```python
from build123d import *

# Parameters (mm, degrees)
SKETCH1_R           = 2.5
BOSS_EXTRUDE1_DEPTH = 10
FILLET1_R           = 20
FILLET2_R           = 2.5


with BuildPart() as part:
    # Sketch1 → Boss-Extrude1 (new body)
    with BuildSketch(Plane(origin=(0, 0, 0), x_dir=(1, 0, 0), z_dir=(0, 1, 0))):
        with BuildLine():
            Line((0, 0), (-300, 0))
            Line((-300, 0), (-300, 125))
            Line((-300, 125), (-287.5, 155))
            Line((-287.5, 155), (-275, 125))
            Line((-275, 125), (-275, 97))
            Line((-275, 97), (-287.66515139, 62))
            ThreePointArc((-287.66515139, 62), (-280.543096437, 48.210936871), (-268.5, 58))
            Line((-268.5, 58), (-268.5, 83))
            ThreePointArc((-268.5, 83), (-262.136038969, 80.363961031), (-259.5, 74))
            Line((-259.5, 74), (-259.5, 25))
            Line((-259.5, 25), (-248.5, 25))
            Line((-248.5, 25), (-248.5, 86.008335649))
            ThreePointArc((-248.5, 86.008335649), (-262.197622342, 96.159801673), (-257.553360344, 112.564311745))
            Line((-257.553360344, 112.564311745), (-242.5, 125))
            Line((-242.5, 125), (-230, 155))
            Line((-230, 155), (-217.5, 125))
            Line((-217.5, 125), (-217.5, 97))
            Line((-217.5, 97), (-230.16515139, 62))
            ThreePointArc((-230.16515139, 62), (-223.043096437, 48.210936871), (-211, 58))
            Line((-211, 58), (-211, 83))
            ThreePointArc((-211, 83), (-204.636038969, 80.363961031), (-202, 74))
            Line((-202, 74), (-202, 25))
            Line((-202, 25), (-191, 25))
            Line((-191, 25), (-191, 86.008335649))
            ThreePointArc((-191, 86.008335649), (-204.697622342, 96.159801673), (-200.053360344, 112.564311745))
            Line((-200.053360344, 112.564311745), (-185, 125))
            Line((-185, 125), (-172.5, 155))
            Line((-172.5, 155), (-160, 125))
            Line((-160, 125), (-160, 97))
            Line((-160, 97), (-172.66515139, 62))
            ThreePointArc((-172.66515139, 62), (-165.543096437, 48.210936871), (-153.5, 58))
            Line((-153.5, 58), (-153.5, 83))
            ThreePointArc((-153.5, 83), (-147.136038969, 80.363961031), (-144.5, 74))
            Line((-144.5, 74), (-144.5, 25))
            Line((-144.5, 25), (-133.5, 25))
            Line((-133.5, 25), (-133.5, 86.008335649))
            ThreePointArc((-133.5, 86.008335649), (-147.197622342, 96.159801673), (-142.553360344, 112.564311745))
            Line((-142.553360344, 112.564311745), (-127.5, 125))
            Line((-127.5, 125), (-115, 155))
            Line((-115, 155), (-102.5, 125))
            Line((-102.5, 125), (-102.5, 97))
            Line((-102.5, 97), (-115.16515139, 62))
            ThreePointArc((-115.16515139, 62), (-108.043096437, 48.210936871), (-96, 58))
            Line((-96, 58), (-96, 83))
            ThreePointArc((-96, 83), (-89.636038969, 80.363961031), (-87, 74))
            Line((-87, 74), (-87, 25))
            Line((-87, 25), (-76, 25))
            Line((-76, 25), (-76, 86.008335649))
            ThreePointArc((-76, 86.008335649), (-89.697622342, 96.159801673), (-85.053360344, 112.564311745))
            Line((-85.053360344, 112.564311745), (-70, 125))
            Line((-70, 125), (-57.5, 155))
            Line((-57.5, 155), (-45, 125))
            Line((-45, 125), (-45, 97))
            Line((-45, 97), (-57.66515139, 62))
            ThreePointArc((-57.66515139, 62), (-50.543096437, 48.210936871), (-38.5, 58))
            Line((-38.5, 58), (-38.5, 83))
            ThreePointArc((-38.5, 83), (-32.136038969, 80.363961031), (-29.5, 74))
            Line((-29.5, 74), (-29.5, 25))
            Line((-29.5, 25), (-18.5, 25))
            Line((-18.5, 25), (-18.5, 86.008335649))
            ThreePointArc((-18.5, 86.008335649), (-32.197622342, 96.159801673), (-27.553360344, 112.564311745))
            Line((-27.553360344, 112.564311745), (-12.5, 125))
            Line((-12.5, 125), (0, 155))
            Line((0, 155), (0, 0))
        make_face()
        with Locations(Location((-5, 125, 0), (0, 0, 270))):
            Circle(SKETCH1_R, mode=Mode.SUBTRACT)
        with Locations(Location((-58.5, 87, 0), (0, 0, 270))):
            Circle(SKETCH1_R, mode=Mode.SUBTRACT)
        with Locations(Location((-62.5, 125, 0), (0, 0, 270))):
            Circle(SKETCH1_R, mode=Mode.SUBTRACT)
        with Locations(Location((-116, 87, 0), (0, 0, 270))):
            Circle(SKETCH1_R, mode=Mode.SUBTRACT)
        with Locations(Location((-120, 125, 0), (0, 0, 270))):
            Circle(SKETCH1_R, mode=Mode.SUBTRACT)
        with Locations(Location((-173.5, 87, 0), (0, 0, 270))):
            Circle(SKETCH1_R, mode=Mode.SUBTRACT)
        with Locations(Location((-177.5, 125, 0), (0, 0, 270))):
            Circle(SKETCH1_R, mode=Mode.SUBTRACT)
        with Locations(Location((-231, 87, 0), (0, 0, 270))):
            Circle(SKETCH1_R, mode=Mode.SUBTRACT)
        with Locations(Location((-235, 125, 0), (0, 0, 270))):
            Circle(SKETCH1_R, mode=Mode.SUBTRACT)
        with Locations(Location((-288.5, 87, 0), (0, 0, 270))):
            Circle(SKETCH1_R, mode=Mode.SUBTRACT)
    extrude(amount=BOSS_EXTRUDE1_DEPTH)

    # Fillet1
    fillet1_edges = [part.edges().sort_by_distance(p)[0] for p in [
        (-275, 5, -125),
        (-275, 5, -97),
        (-248.5, 5, -86.008335649),
        (-242.5, 5, -125),
        (-217.5, 5, -125),
        (-217.5, 5, -97),
        (-191, 5, -86.008335649),
        (-185, 5, -125),
        (-160, 5, -125),
        (-160, 5, -97),
        (-133.5, 5, -86.008335649),
        (-127.5, 5, -125),
        (-102.5, 5, -125),
        (-102.5, 5, -97),
        (-76, 5, -86.008335649),
        (-70, 5, -125),
        (-45, 5, -125),
        (-45, 5, -97),
        (-18.5, 5, -86.008335649),
        (-12.5, 5, -125),
    ]]
    fillet(fillet1_edges, radius=FILLET1_R)

    # Fillet2
    fillet2_edges = [part.edges().sort_by_distance(p)[0] for p in [
        (-268.5, 5, -83),
        (-211, 5, -83),
        (-153.5, 5, -83),
        (-96, 5, -83),
        (-38.5, 5, -83),
    ]]
    fillet(fillet2_edges, radius=FILLET2_R)


solid = part.part
```
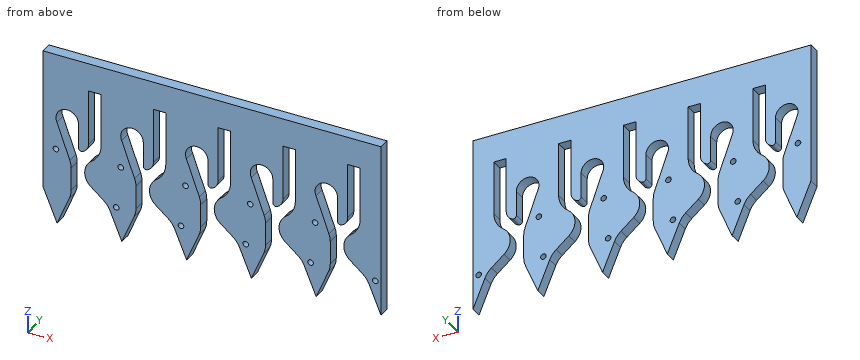
Geometry check sheet. Reference: the model listing, model coordinates, mm. Give positions to 0.01 mm unless a question says otherwise; leave off trailing zeros. Write each question's results on one line, items separated by ' | '. Start each with the question number.
(1) Sectioned sample at A-A (y = 8.5). Give the number of separate pieces and of enclosed holes in the cut face, plus the area to 3 significant figures.
(2) Scan lines: line 1 (X direction, y = 2.25, z = -31); line 2 (Z direction, x = -60.5, y = 3.75); line 3 (X direction, y = 4.25, z = -115). Record each from-to range of solid material in increasing order.
(3) Gauge pin test, flat ends, axial feed: P1, Ø5, axis at x = -194, y = 7, coming from the -Z side; P2, Ø3, axis at x = -223, y = 1.5, coming from the -Z side. Record the tip position at first contact, or that the pin passes through.
Answer below:
1) separate pieces: 1 | enclosed holes: 10 | area: 29,300 mm2
2) line 1: -300 to -259.5, -248.5 to -202, -191 to -144.5, -133.5 to -87, -76 to -29.5, -18.5 to 0 | line 2: -147.8 to -126.5, -123.5 to -88.5, -85.5 to 0 | line 3: -300 to -275, -254.6 to -217.5, -197.1 to -160, -139.6 to -102.5, -82.1 to -45, -24.6 to 0
3) P1: z = -119.63 | P2: z = -141.8
